Geometry check sheet. Reference: the model listing, model coordinates, mm. Give positions to 0.01 mm unless a question says otherwise; leave off trailing zeros. Write each loop counter-clockwise with the first axis right and the second up, starting at its lowest first coordinate (ties: lowest second). Pieces come first, ordered by that corner, then holes. Notation, with made-up numbers: (28, 26) -> (86, 26) arc R14 ccw to (86, 31) -> close; hole circle Ø7 at (57, 6.25). An arc over 180 degrees is marked (long way). Use a Markdown table: item, result. Add a question column.
from build123d import *

# Parameters (mm, degrees)
SKETCH_1_R               = 29.8
SKETCH_1_R_2             = 17.2
EXTRUDE_1_DEPTH          = 1.1
SKETCH_2_R               = 29.5
SKETCH_2_R_2             = 25.5
SKETCH_2_R_3             = 21.5
SKETCH_2_R_4             = 17.5
EXTRUDE_2_DEPTH          = 0.1
SKETCH_4_R               = 0.5
CUT_EXTRUDE_1_DEPTH      = 43.157917406
EXTRUDE_START            = 0.1
SKETCH_5_R               = 1.345948063
SKETCH_5_R_2             = 0.5
EXTRUDE_3_DEPTH          = 0.1
PATTERN_CIRCULAR_1_COUNT = 2
PATTERN_CIRCULAR_1_ANGLE = 10
EXTRUDE_4_DEPTH          = 0.1


with BuildPart() as part:
    # Эскиз1 → Бобышка-Вытянуть1 (new body)
    with BuildSketch(Plane(origin=(0, 0, 0), x_dir=(1, 0, 0), z_dir=(0, 1, 0))):
        with Locations(Location((0, 0, 0), (0, 0, 270))):
            Circle(SKETCH_1_R)
        with Locations(Location((0, 0, 0), (0, 0, 270))):
            Circle(SKETCH_1_R_2, mode=Mode.SUBTRACT)
    extrude(amount=EXTRUDE_1_DEPTH)

    # Эскиз2 → Бобышка-Вытянуть2 (add)
    # profile 1 of 2: a face of its own
    with BuildSketch(Plane(origin=(0, 1.1, 0), x_dir=(1, 0, 0), z_dir=(0, 1, 0))):
        with Locations(Location((0, 0, 0), (0, 0, 270))):
            Circle(SKETCH_2_R)
        with Locations(Location((0, 0, 0), (0, 0, 270))):
            Circle(SKETCH_2_R_2, mode=Mode.SUBTRACT)
    # profile 2 of 2: a face of its own
    with BuildSketch(Plane(origin=(0, 1.1, 0), x_dir=(1, 0, 0), z_dir=(0, 1, 0))):
        with Locations(Location((0, 0, 0), (0, 0, 270))):
            Circle(SKETCH_2_R_3)
        with Locations(Location((0, 0, 0), (0, 0, 270))):
            Circle(SKETCH_2_R_4, mode=Mode.SUBTRACT)
    extrude(amount=EXTRUDE_2_DEPTH)

    # Эскиз4 → Вырез-Вытянуть1 (cut, through all)
    with BuildSketch(Plane(origin=(0, 1.1, 0), x_dir=(1, 0, 0), z_dir=(0, 1, 0))):
        with Locations(Location((-23.5, 0, 0), (0, 0, 270))):
            Circle(SKETCH_4_R)
    cut_extrude_1 = extrude(amount=-CUT_EXTRUDE_1_DEPTH, mode=Mode.SUBTRACT)

    # Эскиз5 → Бобышка-Вытянуть3 (add)
    with BuildSketch(Plane(origin=(0, 1.1, 0), x_dir=(1, 0, 0), z_dir=(0, 1, 0)).offset(EXTRUDE_START)):
        with Locations(Location((-23.5, 0, 0), (0, 0, 270))):
            Circle(SKETCH_5_R)
        with Locations(Location((-23.5, 0, 0), (0, 0, 270))):
            Circle(SKETCH_5_R_2, mode=Mode.SUBTRACT)
    extrude_3 = extrude(amount=-EXTRUDE_3_DEPTH)

    # Круговой массив1: Вырез-Вытянуть1, Бобышка-Вытянуть3 ×2 about axis
    pattern_circular_1_axis = Axis((0, 1.1, 0), (0, -1, 0))
    add([cut_extrude_1.rotate(pattern_circular_1_axis, i * PATTERN_CIRCULAR_1_ANGLE / (PATTERN_CIRCULAR_1_COUNT - 1)) for i in range(1, PATTERN_CIRCULAR_1_COUNT)], mode=Mode.SUBTRACT)
    add([extrude_3.rotate(pattern_circular_1_axis, i * PATTERN_CIRCULAR_1_ANGLE / (PATTERN_CIRCULAR_1_COUNT - 1)) for i in range(1, PATTERN_CIRCULAR_1_COUNT)])

    # Эскиз6 → Бобышка-Вытянуть4 (add)
    with BuildSketch(Plane(origin=(0, 1.1, 0), x_dir=(1, 0, 0), z_dir=(0, 1, 0))):
        with BuildLine():
            Line((-22.800516228, 5.382382378), (-20.899198346, 5.047128736))
            ThreePointArc((-20.899198346, 5.047128736), (-21.165886934, 3.775609923), (-21.355289338, 2.490304658))
            Line((-21.355289338, 2.490304658), (-23.266360042, 2.740450826))
            ThreePointArc((-23.266360042, 2.740450826), (-21.817482108, 3.847010747), (-22.800516228, 5.382382378))
        make_face()
        Polygon((-23.5, -1.345948063), (-27.456522895, -1.345948063), (-27.456522895, 1.345948063), (-23.5, 1.345948063), (-24.412849666, 0), align=None)
    extrude(amount=EXTRUDE_4_DEPTH)


solid = part.part
1) Sectioned sample at C-C, the plane z = 24. Enter the section's corners in (x, y).
2) Material ranges on probe 1 along X at (y, z) = (0.85, 0); probe 2 along X at (y, z) = (0.65, -4.5); probe 3 along Z at (x, y) = (11, 0.65), recorded low to high. Write a range as [from, to].
3) Sectioned sample at A-A, the plane x = 0. Enter the section's corners in (y, z).
4) Sectioned sample at B-B, the plane x = -12. Enter the section's corners in (y, z), and give its area (3 significant figures).
5) Draft check along X on faces 1 (the face through (13.2, 1.2, -22)), 2 (the face through (13.3, 1.1, -17.1)), 3 (the face through (-26.44, 0.54, 13.75)), 4 (the face through (-10.466, 0.542, -13.649)). Enter one of: +X half, -X half, draft (parallel to the pull), parting line (faces both ways), or undercut.
6) Sectioned sample at D-D, the plane x = -18.5. Enter the section's corners in (y, z).
7) Gauge pin test, flat end, axial feed: P1, Ø4, axis at x = -12.5, z = -16, coming from the -Y side. Record the tip position at first contact, or that the pin passes through.
Check values:
| question | item | result |
|---|---|---|
| 1 | outline | (-17.66, 0) -> (17.66, 0) -> (17.66, 1.1) -> (17.15, 1.1) -> (17.15, 1.2) -> (8.62, 1.2) -> (8.62, 1.1) -> (-8.62, 1.1) -> (-8.62, 1.2) -> (-17.15, 1.2) -> (-17.15, 1.1) -> (-17.66, 1.1) -> close |
| 2 | probe 1 | [-29.8, -24], [-23, -17.2], [17.2, 29.8] |
| 2 | probe 2 | [-29.46, -23.42], [-22.87, -16.6], [16.6, 29.46] |
| 2 | probe 3 | [-27.7, -13.22], [13.22, 27.7] |
| 3 | outline | (0, -29.8) -> (1.1, -29.8) -> (1.1, -29.5) -> (1.2, -29.5) -> (1.2, -25.5) -> (1.1, -25.5) -> (1.1, -21.5) -> (1.2, -21.5) -> (1.2, -17.5) -> (1.1, -17.5) -> (1.1, -17.2) -> (0, -17.2) -> close; (0, 17.2) -> (1.1, 17.2) -> (1.1, 17.5) -> (1.2, 17.5) -> (1.2, 21.5) -> (1.1, 21.5) -> (1.1, 25.5) -> (1.2, 25.5) -> (1.2, 29.5) -> (1.1, 29.5) -> (1.1, 29.8) -> (0, 29.8) -> close |
| 4 | outline | (0, -27.28) -> (1.1, -27.28) -> (1.1, -26.95) -> (1.2, -26.95) -> (1.2, -22.5) -> (1.1, -22.5) -> (1.1, -17.84) -> (1.2, -17.84) -> (1.2, -12.74) -> (1.1, -12.74) -> (1.1, -12.32) -> (0, -12.32) -> close; (0, 12.32) -> (1.1, 12.32) -> (1.1, 12.74) -> (1.2, 12.74) -> (1.2, 17.84) -> (1.1, 17.84) -> (1.1, 22.5) -> (1.2, 22.5) -> (1.2, 26.95) -> (1.1, 26.95) -> (1.1, 27.28) -> (0, 27.28) -> close |
| 4 | area | 34.8 mm² |
| 5 | face 1 | draft |
| 5 | face 2 | undercut |
| 5 | face 3 | parting line |
| 5 | face 4 | undercut |
| 6 | outline | (0, -23.36) -> (1.1, -23.36) -> (1.1, -22.98) -> (1.2, -22.98) -> (1.2, -17.55) -> (1.1, -17.55) -> (1.1, -10.95) -> (1.2, -10.95) -> (1.2, 10.95) -> (1.1, 10.95) -> (1.1, 17.55) -> (1.2, 17.55) -> (1.2, 22.98) -> (1.1, 22.98) -> (1.1, 23.36) -> (0, 23.36) -> close |
| 7 | P1 | y = 0 |
